Build history of the part. All positions in model axes, mm. Face numbers are marked on the shaded views. A direction names the side the tool comes from. Round coordinates to 2 decimals unless told otherwise and drop trailing zeros. Write each loop counter-clockwise with the first axis right and the second up, starting at its lowest first coordinate (ties: lowest second). Pieces come first, ordered by that corner, then holes. Notation, with made-up numbers: (-6.75, 55) -> (48.25, 55) arc R32 cw to (48.25, 84) -> close; hole circle Ø10 at (63, -31.75). An arc over 180 degrees is marked (long way). Answer as CSV lines item,"result".
from build123d import *

# Parameters (mm, degrees)
F0_W     = 170
F0_H     = 25
F1_DEPTH = 50
F2_R     = 5
F3_DEPTH = 50.001
F5_DEPTH = 25.001
F7_DEPTH = 25.001
F8_R     = 10


with BuildPart() as f1:
    # F0 (on Top) → F1 (new body)
    with BuildSketch(Plane.XY):
        with Locations((85, 12.5)):
            Rectangle(F0_W, F0_H)
    extrude(amount=F1_DEPTH)

    # F2 (on face) → F3 (cut, through all)
    with BuildSketch(Plane.XY.offset(50)):
        with Locations((11.25, 12.5)):
            Circle(F2_R)
        with Locations((158.75, 12.5)):
            Circle(F2_R)
    extrude(amount=-F3_DEPTH, mode=Mode.SUBTRACT)

    # F4 (on face) → F5 (cut, through all)
    with BuildSketch(Plane.XZ):
        Polygon((100, 31.5), (92.5, 31.5), (92.5, 32.220282), (85, 32.220282), (77.5, 32.220282), (77.5, 31.5), (70, 31.5), (70, 28.694315), (64, 28.694315), (64, 25.794553), (58, 25.794553), (58, 21.515869), (52, 21.515869), (52, 15.164459), (48, 15.164459), (48, 8.794946), (45.5, 8.794946), (45.5, 2.727922), (44.5, 2.727922), (44.5, 0), (125.5, 0), (125.5, 2.727922), (124.5, 2.727922), (124.5, 8.794946), (122, 8.794946), (122, 15.164459), (118, 15.164459), (118, 21.515869), (112, 21.515869), (112, 25.794553), (106, 25.794553), (106, 28.694315), (100, 28.694315), align=None)
    extrude(amount=-F5_DEPTH, mode=Mode.SUBTRACT)

    # F6 (on face) → F7 (cut, through all)
    with BuildSketch(Plane(origin=(0, 25, 0), x_dir=(-1, 0, 0), z_dir=(0, 1, 0))):
        with BuildLine():
            Line((-170, 22), (-144, 22))
            ThreePointArc((-144, 22), (-128.910808, 38.844978), (-109.23843, 50))
            Line((-109.23843, 50), (-170, 50))
            Line((-170, 50), (-170, 22))
        make_face()
        with BuildLine():
            Line((-26, 22), (0, 22))
            Line((0, 22), (0, 50))
            Line((0, 50), (-60.76157, 50))
            ThreePointArc((-60.76157, 50), (-41.089192, 38.844978), (-26, 22))
        make_face()
    extrude(amount=-F7_DEPTH, mode=Mode.SUBTRACT)

    # F8
    f8_edges = [f1.edges().sort_by_distance(p)[0] for p in [
        (144, 12.5, 22),
        (26, 12.5, 22),
    ]]
    fillet(f8_edges, radius=F8_R)


solid = f1.part
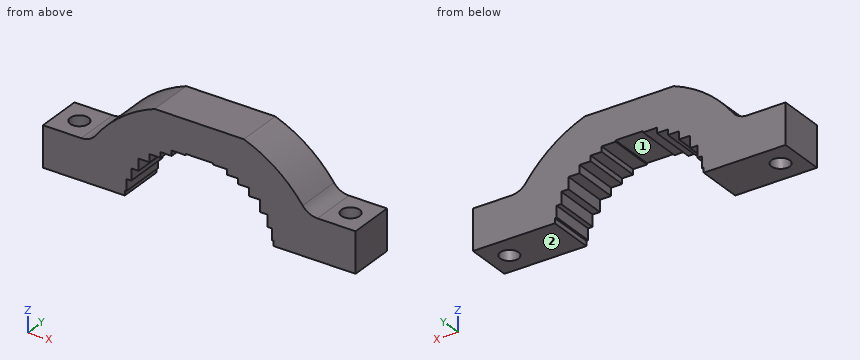
1. Drop flat-ended pins along their axis: pin 1 Ø3 at (x, y) = (123.5, 14.5) entering from -Z; pin 2 Ø8 at (x, y) = (113.5, 4) entering from +Z; pin 3 Ø1.8 at (x, y) = (108, 14.5) entering from -Z; pin 4 Ø0.8 at (y, z) = (13, 1.5) entering from -X. Give the stop position or say it passes through.
Results found:
pin 1,"stops at z = 2.73"
pin 2,"stops at z = 49.9"
pin 3,"stops at z = 25.79"
pin 4,"stops at x = 0"
2. Probe line 1 along Y through (x, z) = (11.25, 16.5); line 2 along X through (y, z) = (1.75, 19); line 3 along X through (y, z) = (23, 8.5). List the from-to ranges inside material, lowest first.
Results found:
line 1,"y = 0 to 7.5, 17.5 to 25"
line 2,"x = 0 to 52, 118 to 170"
line 3,"x = 0 to 45.5, 124.5 to 170"
3. Cut at D-D, the plane y = 12.5. Count the separate pieces of the cut face and the enclosed holes in it, then the cut area to 3 significant figures.
Results found:
separate pieces,"3"
enclosed holes,"0"
area,"3,820 mm2"
4. Cut at C-C, the plane z = 19. Write the cut outline in (x, y), then the cut area to 3 significant figures.
Results found:
outline,"(0, 0) -> (52, 0) -> (52, 25) -> (0, 25) -> close; (118, 0) -> (170, 0) -> (170, 25) -> (118, 25) -> close; hole circle Ø10 at (11.25, 12.5); hole circle Ø10 at (158.75, 12.5)"
area,"2,440 mm2"
5. Cut at B-B, the plane x = 11.25. Write the cut outline in (y, z), then the cut area to 3 significant figures.
Results found:
outline,"(0, 0) -> (7.5, 0) -> (7.5, 22) -> (0, 22) -> close; (17.5, 0) -> (25, 0) -> (25, 22) -> (17.5, 22) -> close"
area,"330 mm2"
6. Cut at A-A, the plane z = 4.5. Write the cut outline in (x, y), then the cut area to 3 significant figures.
Results found:
outline,"(0, 0) -> (45.5, 0) -> (45.5, 25) -> (0, 25) -> close; (124.5, 0) -> (170, 0) -> (170, 25) -> (124.5, 25) -> close; hole circle Ø10 at (11.25, 12.5); hole circle Ø10 at (158.75, 12.5)"
area,"2,120 mm2"
7. Which spindle directions (+Z, -Z, +X, -X, +Y, -Y) get a long thin tool onto all of the face, cutting with end or side? Do the marked faces 1 and 2. Say none if no direction does.
Results found:
face 1,"-Z, +Y, -Y"
face 2,"-Z, +X, -X, +Y, -Y"
